The listing builds one solid part. Answer for the finished solid, in the listing's coordinates (mm). A direction names the side the tool comes from. Give positions to 0.01 mm unless a question says otherwise; leave off trailing zeros. Loops run counter-clockwise (first coordinate to the right, second up) from the corner with the lowest first, then second, coordinate; pieces in that order, holes last.
Item 1: A tool of negligible diameter and unlimited length cuts with its end or side. For faces 3 (the face through (-22.36, 15.24, 1.98)), 4 (the face through (-20.741, 9, 9)), 5 (the face through (16.863, 0, 1)), from which of +Z, -Z, +X, -X, +Y, -Y can it reach the whole face along a straight path? Write none if from no direction.
Item 2: Section B-B, the plane x = -6.5 is taken. Give the vertices of the cut face in (y, z).
Item 3: Section D-D, the plane y = 41 is taken. Give the vertices of the cut face in (x, z).
Item 4: The mould has two halves that part along Y. Classify faces 1 (the face through (-22.26, 26.1, 8.89)), 2 (the face through (0, 2.6, 5)): pulls with the +Y half, pulls with the -Y half, needs draft (parallel to the pull), parting line crosses it, or undercut.
Item 5: Section C-C, the plane x = -13 is taken. Give the vertices of the cut face in (y, z).
Item 6: Section A-A, the plane z = 4.75 is taken. Give the vertices of the cut face in (x, y), and give its area (3 significant figures).
Item 7: Consider line 1 along Y through (x, z) = (-11.5, 8.5); line 2 along X through (y, z) = (36.5, 1); line 3 along X through (y, z) = (1.2, 4.75). Determine where each line is inside the solid, lowest interval first.
Item 8: Each of these flat-tipped pins is pushed along its axis until it touches: pin 1 Ø1 at (y, z) = (0, 0.5) entering from +X; pin 2 Ø1.5 at (x, z) = (-13, 2) entering from +Y; pin 3 Ø1 at (y, z) = (10.5, 9) entering from +X. Where does it stop, or does it pass through?
from build123d import *

# Parameters (mm, degrees)
EXTRUDE_1_DEPTH      = 9.5
SKETCH_2_R           = 3
CUT_EXTRUDE_1_DEPTH  = 66.909407523
SKETCH_4_R           = 3
CUT_EXTRUDE_2_DEPTH  = 53.175568995
FILLET_1_R           = 5
SKETCH_5_W           = 3
SKETCH_5_H           = 7.292258694
SKETCH_5_H_2         = 7.292258695
SKETCH_5_W_2         = 7.292258695
SKETCH_5_H_3         = 3
SKETCH_5_W_3         = 7.292258694
CUT_EXTRUDE_3_DEPTH  = 1.2
CHAMFER_1_SIZE       = 1.2
CHAMFER_2_SIZE       = 1.2
MIRROR_START         = -23.741274046
MIRROR_1_OUTLINE_W   = 7.292258694
MIRROR_1_OUTLINE_H   = 1.2
MIRROR_1_OUTLINE_W_2 = 7.292258695
MIRROR_1_DEPTH       = 3
MIRROR_START_2       = -16.84868645
MIRROR_1_2_OUTLINE_W = 3
MIRROR_1_2_OUTLINE_H = 1.2
MIRROR_1_2_DEPTH     = 7.292258695
MIRROR_START_3       = -4.181235969
MIRROR_1_3_OUTLINE_W = 3
MIRROR_1_3_OUTLINE_H = 1.2
MIRROR_1_3_DEPTH     = 7.292258694
MIRROR_START_4       = 9.571089537
MIRROR_1_4_OUTLINE_W = 3
MIRROR_1_4_OUTLINE_H = 1.2
MIRROR_1_4_DEPTH     = 7.292258694


# Read off the part's stored shape, not the designer's step: 镜向1
with BuildPart() as part:
    # 草图1 → 凸台-拉伸1 (new body)
    with BuildSketch(Plane.XY):
        Polygon((-19.8, 2.6), (-19.8, 47.4), (-25, 47.4), (-25, -2.6), (25, -2.6), (25, 2.6), align=None)
    extrude(amount=EXTRUDE_1_DEPTH)

    # 草图2 → 切除-拉伸1 (cut, through all)
    with BuildSketch(Plane(origin=(-19.8, 0, 0), x_dir=(0, 0, -1), z_dir=(1, 0, 0))):
        with Locations((-4.75, 32.604835918)):
            Circle(SKETCH_2_R)
        with Locations((-4.75, 16.388429447)):
            Circle(SKETCH_2_R)
    extrude(amount=-CUT_EXTRUDE_1_DEPTH, mode=Mode.SUBTRACT)

    # 草图4 → 切除-拉伸2 (cut, through all)
    with BuildSketch(Plane(origin=(0, 2.6, 0), x_dir=(1, 0, 0), z_dir=(0, 1, 0))):
        with Locations(Location((9.252806551, -4.75, 0), (0, 0, 270))):
            Circle(SKETCH_4_R)
        with Locations(Location((-5.859043595, -4.75, 0), (0, 0, 270))):
            Circle(SKETCH_4_R)
    extrude(amount=-CUT_EXTRUDE_2_DEPTH, mode=Mode.SUBTRACT)

    # 圆角1
    fillet_1_edges = [part.edges().sort_by_distance(p)[0] for p in [
        (-19.8, 47.4, 4.75),
        (25, 2.6, 4.75),
    ]]
    fillet(fillet_1_edges, radius=FILLET_1_R)

    # 草图5 → 切除-拉伸3 (cut)
    with BuildSketch(Plane.XY.offset(9.5)):
        with Locations((-22.241274046, 21.864893378)):
            Rectangle(SKETCH_5_W, SKETCH_5_H)
        with Locations((-22.241274046, 35.617218884)):
            Rectangle(SKETCH_5_W, SKETCH_5_H)
        with Locations((-22.241274046, 9.197442898)):
            Rectangle(SKETCH_5_W, SKETCH_5_H_2)
        with Locations((-13.202557103, 0.158725954)):
            Rectangle(SKETCH_5_W_2, SKETCH_5_H_3)
        with Locations((-0.535106622, 0.158725954)):
            Rectangle(SKETCH_5_W_3, SKETCH_5_H_3)
        with Locations((13.217218884, 0.158725954)):
            Rectangle(SKETCH_5_W_3, SKETCH_5_H_3)
    extrude(amount=-CUT_EXTRUDE_3_DEPTH, mode=Mode.SUBTRACT)

    # 倒角1
    chamfer_1_edges = [part.edges().sort_by_distance(p)[0] for p in [
        (-22.241274046, 5.55131355, 9.5),
        (-22.241274046, 12.843572245, 9.5),
        (-22.241274046, 18.218764031, 9.5),
        (-22.241274046, 25.511022725, 9.5),
        (-22.241274046, 39.263348231, 8.3),
        (-22.241274046, 31.971089537, 9.5),
    ]]
    chamfer(chamfer_1_edges, length=CHAMFER_1_SIZE - 0.0001)  # a hair under: the kernel refuses the full size

    # 倒角2
    chamfer_2_edges = [part.edges().sort_by_distance(p)[0] for p in [
        (16.863348231, 0.158725954, 9.5),
        (9.571089537, 0.158725954, 9.5),
        (3.111022725, 0.158725954, 9.5),
        (-4.181235969, 0.158725954, 9.5),
        (-9.556427755, 0.158725954, 9.5),
        (-16.84868645, 0.158725954, 9.5),
    ]]
    chamfer(chamfer_2_edges, length=CHAMFER_2_SIZE - 0.0001)  # a hair under: the kernel refuses the full size

    # 镜向1 outline → 镜向1 (cut)
    with BuildSketch(Plane.YZ.offset(MIRROR_START)):
        Polygon((31.971089537, 1.2), (31.971089537, 0), (39.263348231, 0), (38.063348231, 1.2), align=None)
        with Locations((21.864893378, 0.6)):
            Rectangle(MIRROR_1_OUTLINE_W, MIRROR_1_OUTLINE_H)
        with Locations((9.197442898, 0.6)):
            Rectangle(MIRROR_1_OUTLINE_W_2, MIRROR_1_OUTLINE_H)
    extrude(amount=MIRROR_1_DEPTH, mode=Mode.SUBTRACT)

    # Mirror 1 2 outline → Mirror 1 2 (cut)
    with BuildSketch(Plane.YZ.offset(MIRROR_START_2)):
        with Locations((0.158725954, 0.6)):
            Rectangle(MIRROR_1_2_OUTLINE_W, MIRROR_1_2_OUTLINE_H)
    extrude(amount=MIRROR_1_2_DEPTH, mode=Mode.SUBTRACT)

    # Mirror 1 3 outline → Mirror 1 3 (cut)
    with BuildSketch(Plane.YZ.offset(MIRROR_START_3)):
        with Locations((0.158725954, 0.6)):
            Rectangle(MIRROR_1_3_OUTLINE_W, MIRROR_1_3_OUTLINE_H)
    extrude(amount=MIRROR_1_3_DEPTH, mode=Mode.SUBTRACT)

    # Mirror 1 4 outline → Mirror 1 4 (cut)
    with BuildSketch(Plane.YZ.offset(MIRROR_START_4)):
        with Locations((0.158725954, 0.6)):
            Rectangle(MIRROR_1_4_OUTLINE_W, MIRROR_1_4_OUTLINE_H)
    extrude(amount=MIRROR_1_4_DEPTH, mode=Mode.SUBTRACT)


solid = part.part
Worked answers:
1. face 3: +X, -X
1. face 4: +Z
1. face 5: -Z
2. outline: (-2.6, 0) - (2.6, 0) - (2.6, 1.82) - (-2.6, 1.82) - close; (-2.6, 7.68) - (2.6, 7.68) - (2.6, 9.5) - (-2.6, 9.5) - close
3. outline: (-25, 0) - (-19.8, 0) - (-19.8, 9.5) - (-25, 9.5) - close
4. face 1: undercut
4. face 2: pulls with the +Y half
5. outline: (-2.6, 0) - (-1.34, 0) - (-1.34, 1.2) - (1.66, 1.2) - (1.66, 0) - (2.6, 0) - (2.6, 9.5) - (1.66, 9.5) - (1.66, 8.3) - (-1.34, 8.3) - (-1.34, 9.5) - (-2.6, 9.5) - close
6. outline: (-25, -2.6) - (-8.86, -2.6) - (-8.86, 2.6) - (-19.8, 2.6) - (-19.8, 13.39) - (-25, 13.39) - close; (-25, 19.39) - (-19.8, 19.39) - (-19.8, 29.6) - (-25, 29.6) - close; (-25, 35.6) - (-19.8, 35.6) - (-19.8, 42.4) arc R5 ccw to (-24.8, 47.4) - (-25, 47.4) - close; (-2.86, -2.6) - (6.25, -2.6) - (6.25, 2.6) - (-2.86, 2.6) - close; (12.25, -2.6) - (25, -2.6) - (25, -2.4) arc R5 ccw to (20, 2.6) - (12.25, 2.6) - close
6. area: 357 mm2
7. line 1: y = -2.6 to -1.34, 1.66 to 2.6
7. line 2: x = -25 to -23.74, -20.74 to -19.8
7. line 3: x = -25 to -8.86, -2.86 to 6.25, 12.25 to 23.47
8. pin 1: stops at x = 24.62
8. pin 2: stops at y = 2.6
8. pin 3: stops at x = -19.8
